Build history of the part. All positions in model axes, mm. Face numbers are marked on the shaded views. A direction names the side the tool comes from. Coordinates: 2 decimals unless noted, no trailing zeros. Order: outer loops, then holes, each group sorted by start corner. A loop starts at its lowest first (then second) coordinate and runs counter-clockwise, first axis right, second up. Notation, with made-up numbers: (68, -17) - (107, -17) arc R22 cw to (107, 1) - close; hole circle Ø2 at (-16, 88.25). An arc over 180 degrees is marked (long way). Write each question's results on one line, items separated by ' | '.
from build123d import *

# Parameters (mm, degrees)
F1_DEPTH     = 75
F2_W         = 21
F2_H         = 75
F3_DEPTH     = 28
F5_DEPTH     = 50.8
F6_W         = 19
F6_H         = 77
F7_DEPTH     = 75
F9_DEPTH     = 38.6
F11_DEPTH    = 19
F12_W        = 19
F12_H        = 77
F13_DEPTH    = 77
F14_W        = 19
F14_H        = 9.9398646951
F15_DEPTH    = 77
F17_DEPTH    = 75.4
F18_T1_DEPTH = 19
F19_T1_DEPTH = 102.8939212925
F19_T3_DEPTH = 186.7878425849


# Not quite as in the source:
# - a fillet or chamfer that OpenCascade refuses, or shapes differently, is made with other operations: its cross-section is extruded or revolved along the edge and cut away or added


with BuildPart() as f1:
    # F0 (on Right) → F1 (new body)
    with BuildSketch(Plane.YZ):
        Polygon((0, 75), (0, 0), (63, 0), (63, 20), (25, 20), (25, 55), (63, 55), (63, 75), align=None)
    extrude(amount=F1_DEPTH)

    # F2 (on face) → F3 (join)
    with BuildSketch(Plane.XZ):
        with Locations((37.5, 37.5)):
            Rectangle(F2_W, F2_H)
    extrude(amount=F3_DEPTH)

    # F4 (on face) → F5 (cut)
    with BuildSketch(Plane(origin=(27, 0, 0), x_dir=(0, -1, 0), z_dir=(-1, 0, 0))):
        Polygon((28, 67), (28, 75), (0, 75), align=None)
    extrude(amount=-F5_DEPTH, mode=Mode.SUBTRACT)

    # F6 (on Top) → F7 (join)
    with BuildSketch(Plane.XY):
        with Locations((57.8057536185, -38.5)):
            Rectangle(F6_W, F6_H)
    extrude(amount=F7_DEPTH)

    # F8 (on face) → F9 (cut)
    with BuildSketch(Plane(origin=(48.3057536185, 0, 0), x_dir=(0, -1, 0), z_dir=(-1, 0, 0))):
        Polygon((77, 75), (0, 75), (27.784453705, 67), (77, 67), align=None)
    extrude(amount=-F9_DEPTH, mode=Mode.SUBTRACT)

    # F10 (on face) → F11 (cut)
    with BuildSketch(Plane.YZ.offset(67.3057536185)):
        Polygon((0, 75), (-27.784453705, 67), (0, 67), align=None)
    extrude(amount=-F11_DEPTH, mode=Mode.SUBTRACT)

    # F12 (on Top) → F13 (join)
    with BuildSketch(Plane.XY):
        with Locations((17.5, -38.5)):
            Rectangle(F12_W, F12_H)
    extrude(amount=F13_DEPTH)

    # F14 (on face) → F15 (cut)
    with BuildSketch(Plane.XZ.offset(77)):
        with Locations((17.5, 72.0300676525)):
            Rectangle(F14_W, F14_H)
    extrude(amount=-F15_DEPTH, mode=Mode.SUBTRACT)

    # F16 (on face) → F17 (cut)
    with BuildSketch(Plane(origin=(8, 0, 0), x_dir=(0, -1, 0), z_dir=(-1, 0, 0))):
        with BuildLine():
            ThreePointArc((57.5, 32), (36.1611652352, 40.8388347648), (45, 19.5))
            ThreePointArc((45, 19.5), (53.8388347648, 23.1611652352), (57.5, 32))
        make_face()
    extrude(amount=-F17_DEPTH, mode=Mode.SUBTRACT)

    # F18: fillet of radius 34.5232539419 on 2 edges, made by hand

    # F18_s2 → F18_t1 (cut)
    with BuildSketch(Plane.YZ.offset(8)):
        with BuildLine():
            ThreePointArc((-42.4767460581, 67.0601353049), (-66.888373029, 56.948508334), (-77, 32.536881363))
            Line((-77, 32.536881363), (-77.6904650788, 32.536881363))
            Line((-77.6904650788, 32.536881363), (-77.6904650788, 67.7506003838))
            Line((-77.6904650788, 67.7506003838), (-42.4767460581, 67.7506003838))
            Line((-42.4767460581, 67.7506003838), (-42.4767460581, 67.0601353049))
        make_face()
        with BuildLine():
            ThreePointArc((-42.4767460581, 0), (-66.888373029, 10.111626971), (-77, 34.5232539419))
            Line((-77, 34.5232539419), (-77.6904650788, 34.5232539419))
            Line((-77.6904650788, 34.5232539419), (-77.6904650788, -0.6904650788))
            Line((-77.6904650788, -0.6904650788), (-42.4767460581, -0.6904650788))
            Line((-42.4767460581, -0.6904650788), (-42.4767460581, 0))
        make_face()
    extrude(amount=F18_T1_DEPTH, mode=Mode.SUBTRACT)

    # F19: fillet of radius 33.557568517 on 2 edges, made by hand

    # F19_s2 → F19_t1 (cut)
    with BuildSketch(Plane.YZ.offset(48.3057536185)):
        with BuildLine():
            ThreePointArc((-77, 33.442431483), (-67.1712157415, 57.1712157415), (-43.442431483, 67))
            Line((-43.442431483, 67), (-77, 67))
            Line((-77, 67), (-77, 33.442431483))
        make_face()
    extrude(amount=F19_T1_DEPTH, mode=Mode.SUBTRACT)

    # F19_s4 → F19_t3 (cut)
    with BuildSketch(Plane.YZ.offset(-35.588167674)):
        with BuildLine():
            ThreePointArc((-43.442431483, 0), (-67.1712157415, 9.8287842585), (-77, 33.557568517))
            Line((-77, 33.557568517), (-77, 0))
            Line((-77, 0), (-43.442431483, 0))
        make_face()
    extrude(amount=F19_T3_DEPTH, mode=Mode.SUBTRACT)


solid = f1.part
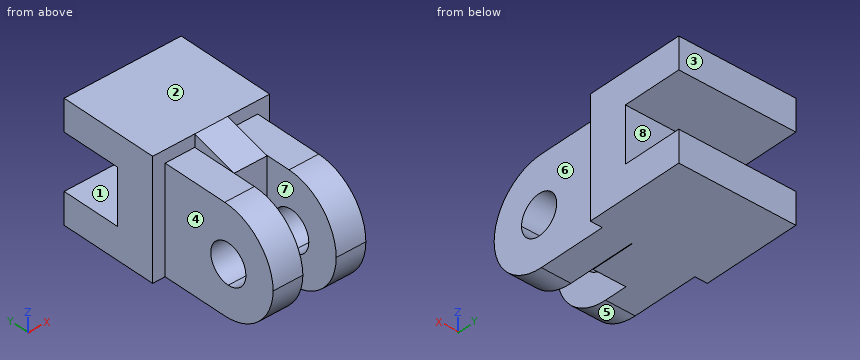
1. Band-saw the part on D-D on z = 16. Give the cut face in (x, y).
Solved:
outline: (0, 0) - (8, 0) - (8, -71.61) - (27, -71.61) - (27, -28) - (48, -28) - (48, 0) - (48.31, 0) - (48.31, -72.04) - (67.31, -72.04) - (67.31, 0) - (75, 0) - (75, 63) - (0, 63) - close
2. Two-plate mould, pull along Z, no slides. Class the marked faces 1, 2 and 3: +Z half, -Z half, draft (parallel to the pull), parting line (faces both ways), or undercut.
Solved:
face 1: undercut | face 2: +Z half | face 3: draft
3. Band-saw the part on C-C on x = 23. Give the cut face in (y, z), then the cut area to 3 significant figures.
Solved:
outline: (-76.99, 33.53) arc R34.52 ccw to (-42.48, 0) - (63, 0) - (63, 20) - (25, 20) - (25, 55) - (63, 55) - (63, 75) - (0, 75) - (0, 67.06) - (-42.48, 67.06) arc R34.52 ccw to start; hole circle Ø25 at (-45, 32) | area: 7,560 mm2
4. Tool access for the marked faces 4, 5, 6, 7 and 8: list every direction of +Z, -Z, +X, -X, +Y, -Y with a clear straight run to the whole face (end or side of a thin tool).
Solved:
face 4: +Z, -Z, -X, -Y | face 5: -Z, -X, -Y | face 6: +Z, -Z, +X, -Y | face 7: +Z, -Z, -Y | face 8: +X, -X, +Y
5. Band-saw the part on A-A on x = 32.5. Give the cut face in (y, z), then the cut area to 3 significant figures.
Solved:
outline: (-28, 0) - (63, 0) - (63, 20) - (25, 20) - (25, 55) - (63, 55) - (63, 75) - (0, 75) - (-28, 67) - close | area: 5,380 mm2
6. Band-saw the part on B-B on y = -8. Give the cut face in (x, z), then the cut area to 3 significant figures.
Solved:
outline: (8, 0) - (48, 0) - (48, 72.71) - (27, 72.71) - (27, 67.06) - (8, 67.06) - close; (48.31, 0) - (67.31, 0) - (67.31, 67) - (48.31, 67) - close | area: 4,070 mm2
7. Probe line 1 (X direction, y = -30.5, z = 34); line 2 (Z direction, x = 19.5, y = 57.5); line 3 (X direction, y = -0.5, z = 36). List the from-to ranges inside material, lowest first.
Solved:
line 1: x = 8 to 27, 48.31 to 67.31 | line 2: z = 0 to 20, 55 to 75 | line 3: x = 8 to 48, 48.31 to 67.31
8. Drop flat-ended pins along their axis: pin 1 Ø3 at (y, z) = (-4.5, 28) entering from -X; pin 2 Ø14 at (y, z) = (-9.5, 50.5) entering from +X; pin 3 Ø8 at (x, z) = (16, 41.5) entering from -Y; pin 4 Ø20 at (y, z) = (-45, 32) entering from -X. Give the stop position or say it passes through.
Solved:
pin 1: stops at x = 8 | pin 2: stops at x = 67.31 | pin 3: stops at y = -76.64 | pin 4: passes through
